Design review of the part built by this model. Coordinates are the model's own, in mm. A direction names the side the tool comes from. Give positions to 0.01 mm unless a question says otherwise; leave off trailing zeros. Loops run counter-clockwise (first coordinate to the right, second up) from the corner with the lowest first, then second, coordinate; pieces in that order, holes last. Notation, with made-up numbers: M -8,-3.75 L 23,-3.75 A20 cw 23,24.25 Z; hole C -4,20 d2. An arc over 180 degrees is marked long. Use a Markdown table: item, result. Add a question column.
(1) Add section A-A, the plane y = 39. Give the boundary of the cut face in (x, z), then the cut area to 3 significant figures.
(2) For probe 1 along X at (y, z) = (-2.5, 26); probe 2 along Z at (x, y) = (19, 0.5); probe 3 along X at (y, z) = (32, 16.5), list the stretches that pass through material, from the lowest coordinate up.
(3) For faces 4 (the face through (8.272, 10, 27)), 5 (the face through (-17, -2.256, 27)), 6 (the face through (-4, -52.789, 27)), list the 3-axis set-ups (+Z, -Z, +X, -X, +Y, -Y) from which the entire face can be reached by the end or side of a thin tool; tool diameter is ignored.
(4) Insertion check: pin 1 Ø10 at (x, y) = (-26.02, 32.03) entering from -Z; pin 2 Ø10 at (x, z) = (21, 20.5) entering from +Y; pin 3 Ø0.8 at (x, z) = (-28.5, 26.5) entering from +Y; pin 4 Ø22 at (x, y) = (-4.89, 19.78) entering from +Z. Each pin has a flat end and moves straight along its axis. Give the tip position at first contact, or say it passes through.
(5) Add section B-B, the plane x = 10.5. Give the boundary of the cut face in (y, z).
(6) Draft analysis for pull direction Y (two halves, no side actions). For faces 1 (the face through (-12, -22.71, 27)), 2 (the face through (-5.201, -58.204, 12.522)), 3 (the face through (-8.272, -48, 27)), state which applies: pulls with the +Y half, pulls with the -Y half, needs draft (parallel to the pull), parting line crosses it, or undercut.
(7) Add section C-C, the plane y = -44. Give the boundary of the cut face in (x, z).
(8) Add section D-D, the plane z = 19.25. Give the boundary of the cut face in (x, y), then the cut area to 3 significant figures.
```python
from build123d import *

# Parameters (mm, degrees)
F1_DEPTH = 19.05
F2_R     = 8.1268855098
F2_R_2   = 8.0990060786
F2_R_3   = 7.6686570694
F2_R_4   = 17.6929682903
F3_DEPTH = 3.81
F4_DEPTH = 6.35
F5_W     = 15.3402648866
F5_H     = 15.9418415278
F5_W_2   = 11.7307901382
F5_H_2   = 14.437895501
F5_W_3   = 12.0315793902
F5_H_3   = 14.1371053178
F5_W_4   = 7.8148348501
F5_H_4   = 12.6331597567
F5_W_5   = 8.2717118785
F5_H_5   = 10.226842016
F5_W_6   = 6.1604853713
F5_H_6   = 12.9339471459
F5_W_7   = 12.4827632681
F5_H_7   = 16.393026337
F5_W_8   = 10.8284177259
F5_H_8   = 14.1371043865
F5_W_9   = 15.6410494819
F5_H_9   = 16.9490305329
F6_DEPTH = 2.54


with BuildPart() as f1:
    # F0 (on Top) → F1 (new body)
    with BuildSketch(Plane.XY):
        with BuildLine():
            ThreePointArc((-13.5217250534, 23.8079438364), (-11.6865877588, 27.7403908158), (-11.0572251912, 32.0340804756))
            ThreePointArc((-11.0572251912, 32.0340804756), (-28.416960574, 46.8016068241), (-40.2102085436, 27.2987980688))
            ThreePointArc((-40.2102085436, 27.2987980688), (-27.9586692008, 17.1993784674), (-13.5217250534, 23.8079438364))
        make_face()
        with BuildLine():
            ThreePointArc((-13.5217250534, 23.8079438364), (-27.9586692008, 17.1993784674), (-40.2102085436, 27.2987980688))
            Line((-40.2102085436, 27.2987980688), (-16.0865467286, -47.5395652548))
            ThreePointArc((-16.0865467286, -47.5395652548), (-12.9985133333, -39.3676590618), (-4.963026382, -35.9402766009))
            Line((-4.963026382, -35.9402766009), (-4.963026382, 10.2515674402))
            ThreePointArc((-4.963026382, 10.2515674402), (-12.9451700449, 14.6920290982), (-13.5217250534, 23.8079438364))
        make_face()
        with BuildLine():
            Line((-14.2646919421, -53.1914696578), (-16.0865467286, -47.5395652548))
            ThreePointArc((-16.0865467286, -47.5395652548), (-15.5593965471, -50.4892255554), (-14.2646919421, -53.1914696578))
        make_face()
        with BuildLine():
            ThreePointArc((-4.963026382, -35.9402766009), (-12.9985133333, -39.3676590618), (-16.0865467286, -47.5395652548))
            Line((-16.0865467286, -47.5395652548), (-14.2646919421, -53.1914696578))
            ThreePointArc((-14.2646919421, -53.1914696578), (-4.963026382, -58.2068318943), (4.3386391781, -53.1914696578))
            Line((4.3386391781, -53.1914696578), (6.1604853713, -47.5397703272))
            ThreePointArc((6.1604853713, -47.5397703272), (6.1678095236, -47.3067134237), (6.1702512647, -47.0735542476))
            ThreePointArc((6.1702512647, -47.0735542476), (2.9093897388, -39.2011381268), (-4.963026382, -35.9402766009))
        make_face()
        with BuildLine():
            ThreePointArc((3.9810605477, 23.2504104806), (2.9582476584, 14.377684043), (-4.963026382, 10.2515674402))
            Line((-4.963026382, 10.2515674402), (-4.963026382, -35.9402766009))
            ThreePointArc((-4.963026382, -35.9402766009), (2.9093897388, -39.2011381268), (6.1702512647, -47.0735542476))
            ThreePointArc((6.1702512647, -47.0735542476), (6.1678095236, -47.3067134237), (6.1604853713, -47.5397703272))
            Line((6.1604853713, -47.5397703272), (30.331755145, 27.443919136))
            ThreePointArc((30.331755145, 27.443919136), (18.4435852345, 17.2589453635), (3.9810605477, 23.2504104806))
        make_face()
        with BuildLine():
            ThreePointArc((31.0533017431, 32.0340804756), (11.4750214501, 46.2648490943), (3.9810605477, 23.2504104806))
            ThreePointArc((3.9810605477, 23.2504104806), (18.4435852345, 17.2589453635), (30.331755145, 27.443919136))
            ThreePointArc((30.331755145, 27.443919136), (30.8718143134, 29.7108171125), (31.0533017431, 32.0340804756))
        make_face()
        with BuildLine():
            Line((6.1604853713, -47.5397703272), (4.3386391781, -53.1914696578))
            ThreePointArc((4.3386391781, -53.1914696578), (5.6333122971, -50.4893232323), (6.1604853713, -47.5397703272))
        make_face()
    extrude(amount=F1_DEPTH)

    # F2 (on face) → F3 (cut)
    with BuildSketch(Plane(origin=(0, 0, 0), x_dir=(1, 0, 0), z_dir=(0, 0, -1))):
        with Locations((-26.0182898492, -32.0340804756)):
            Circle(F2_R)
        with Locations((16.0922370851, -32.0340804756)):
            Circle(F2_R_2)
        with Locations((-4.963026382, 47.0735542476)):
            Circle(F2_R_3)
        with Locations((-5.263815634, 11.279605329)):
            Circle(F2_R_4)
    extrude(amount=-F3_DEPTH, mode=Mode.SUBTRACT)

    # F4 (add): a face of the model
    f4_faces = [f1.faces().sort_by_distance(p)[0] for p in [
        (-4.9663739945, 1.7972425915, 19.05),
    ]]
    extrude(f4_faces, amount=F4_DEPTH)

    # F5 (on face) → F6 (join)
    with BuildSketch(Plane.XY.offset(25.4)):
        with Locations((-26.1686835438, 32.4852624908)):
            Rectangle(F5_W, F5_H)
        with Locations((-24.3639461696, 10.6780267088)):
            Rectangle(F5_W_2, F5_H_2)
        with Locations((-17.2953950241, -9.3244736781)):
            Rectangle(F5_W_3, F5_H_3)
        with Locations((-12.1791293035, -29.026184231)):
            Rectangle(F5_W_4, F5_H_4)
        with Locations((-4.1358559392, -47.6751308888)):
            Rectangle(F5_W_5, F5_H_5)
        with Locations((3.0802426856, -28.8757905364)):
            Rectangle(F5_W_6, F5_H_6)
        with Locations((6.241381634, -8.1965131685)):
            Rectangle(F5_W_7, F5_H_7)
        with Locations((13.6859207414, 10.5276311515)):
            Rectangle(F5_W_8, F5_H_8)
        with Locations((16.3930258714, 32.2824591028)):
            Rectangle(F5_W_9, F5_H_9)
    extrude(amount=F6_DEPTH)


solid = f1.part
```
Established:
| question | item | result |
|---|---|---|
| 1 | outline | M -39.26,0 L -30.2,0 L -30.2,3.81 L -21.83,3.81 L -21.83,0 L -12.78,0 L -12.78,25.4 L -18.5,25.4 L -18.5,27.94 L -33.84,27.94 L -33.84,25.4 L -39.26,25.4 Z; M 2.85,0 L 11.96,0 L 11.96,3.81 L 20.22,3.81 L 20.22,0 L 29.33,0 L 29.33,25.4 L 24.21,25.4 L 24.21,27.94 L 8.57,27.94 L 8.57,25.4 L 2.85,25.4 Z |
| 1 | area | 1,360 mm^2 |
| 2 | probe 1 | -23.31 to -11.28, 0 to 12.48 |
| 2 | probe 2 | 0 to 25.4 |
| 2 | probe 3 | -40.98 to -11.06, 1.13 to 31.05 |
| 3 | face 4 | +Z, +Y |
| 3 | face 5 | +Z, -X |
| 3 | face 6 | +Z, +X, -X, -Y |
| 4 | pin 1 | z = 3.81 |
| 4 | pin 2 | y = 47 |
| 4 | pin 3 | y = 40.46 |
| 4 | pin 4 | z = 25.4 |
| 5 | outline | M -34.08,0 L -19.31,0 L -19.31,3.81 L -3.25,3.81 L -3.25,0 L 26.18,0 L 26.18,3.81 L 37.89,3.81 L 37.89,0 L 45.91,0 L 45.91,25.4 L 40.76,25.4 L 40.76,27.94 L 23.81,27.94 L 23.81,25.4 L 17.6,25.4 L 17.6,27.94 L 3.46,27.94 L 3.46,25.4 L 0,25.4 L 0,27.94 L -16.39,27.94 L -16.39,25.4 L -34.08,25.4 Z |
| 6 | face 1 | undercut |
| 6 | face 2 | pulls with the -Y half |
| 6 | face 3 | needs draft |
| 7 | outline | M -17.23,0 L -11.99,0 L -11.99,3.81 L 2.06,3.81 L 2.06,0 L 7.3,0 L 7.3,25.4 L 0,25.4 L 0,27.94 L -8.27,27.94 L -8.27,25.4 L -17.23,25.4 Z |
| 8 | outline | M -40.21,27.3 L -16.09,-47.54 A11.13 ccw 6.16,-47.54 L 30.33,27.44 A14.96 ccw long 3.98,23.25 A9.53 cw long -13.52,23.81 A14.96 ccw long Z |
| 8 | area | 4,370 mm^2 |
